```python
from build123d import *

# Parameters (mm, degrees)
RESSALTO_EXTRUS_O1_DEPTH = 3
FILETE1_SIZE             = 3.5
FILETE1_SIZE_2           = 2
ESBO_O2_R                = 0.5
RESSALTO_EXTRUS_O4_DEPTH = 0.6
ESBO_O3_R                = 0.5
RESSALTO_EXTRUS_O5_DEPTH = 0.4
FILETE2_R                = 0.2
FILETE2_OF_ESPELHAR1_R   = 0.2
ESBO_O4_R                = 0.4
CORTE_EXTRUS_O1_DEPTH    = 8.735632008


with BuildPart() as part:
    # Esboço1 → Ressalto-extrusão1 (new, symmetric)
    with BuildSketch(Plane(origin=(0, 0, 0), x_dir=(0, 0, -1), z_dir=(1, 0, 0))):
        Polygon((0, 0), (4, 0), (4, -2.8), (-3, -2.8), (-3, -1.8), (2.5, -1.8), (2.5, -1), (0, -1), align=None)
    extrude(amount=RESSALTO_EXTRUS_O1_DEPTH, both=True)

    # Filete1
    # an asymmetric fillet: 3.5, 2 mm, written as the material it takes off along each edge
    with BuildSketch(Plane(origin=(11.75, -2.8, -4), x_dir=(0, 0, 1), z_dir=(-1, 0, 0))) as filete1_piece_1:
        with BuildLine():
            Bezier((FILETE1_SIZE, 0), (0, 0), (0, FILETE1_SIZE_2), weights=[1, 0.707106781, 1])
            Line((0, FILETE1_SIZE_2), (0, 0))
            Line((0, 0), (FILETE1_SIZE, 0))
        make_face()
    extrude(amount=23.5, mode=Mode.SUBTRACT)

    # Esboço2 → Ressalto-extrusão4 (add)
    with BuildSketch(Plane(origin=(0, -1.8, 0), x_dir=(1, 0, 0), z_dir=(0, 1, 0))):
        with Locations(Location((-2, -2, 0), (0, 0, 90))):
            Circle(ESBO_O2_R)
    ressalto_extrus_o4 = extrude(amount=RESSALTO_EXTRUS_O4_DEPTH)

    # Esboço3 → Ressalto-extrusão5 (add)
    with BuildSketch(Plane.XZ.offset(1)):
        with Locations(Location((-2, -1, 0), (0, 0, 90))):
            Circle(ESBO_O3_R)
    ressalto_extrus_o5 = extrude(amount=RESSALTO_EXTRUS_O5_DEPTH)

    # Filete2
    filete2_edges = [part.edges().sort_by_distance(p)[0] for p in [
        (-2, -1.2, 2.5),
        (-2, -1.4, -1.5),
    ]]
    fillet(filete2_edges, radius=FILETE2_R)

    # Espelhar1: Ressalto-extrusão4, Ressalto-extrusão5 across plane
    add(ressalto_extrus_o4.mirror(Plane(origin=(0, 0, 0), x_dir=(0, 0, 1), z_dir=(1, 0, 0))))
    add(ressalto_extrus_o5.mirror(Plane(origin=(0, 0, 0), x_dir=(0, 0, 1), z_dir=(1, 0, 0))))

    # Filete2 of Espelhar1
    filete2_of_espelhar1_edges = [part.edges().sort_by_distance(p)[0] for p in [
        (2, -1.2, 2.5),
        (2, -1.4, -1.5),
    ]]
    fillet(filete2_of_espelhar1_edges, radius=FILETE2_OF_ESPELHAR1_R)

    # Esboço4 → Corte-extrusão1 (cut, through all)
    with BuildSketch(Plane.ZY.offset(3)):
        with Locations((-2.5, -1.4)):
            Circle(ESBO_O4_R)
    extrude(amount=-CORTE_EXTRUS_O1_DEPTH, mode=Mode.SUBTRACT)


solid = part.part
```
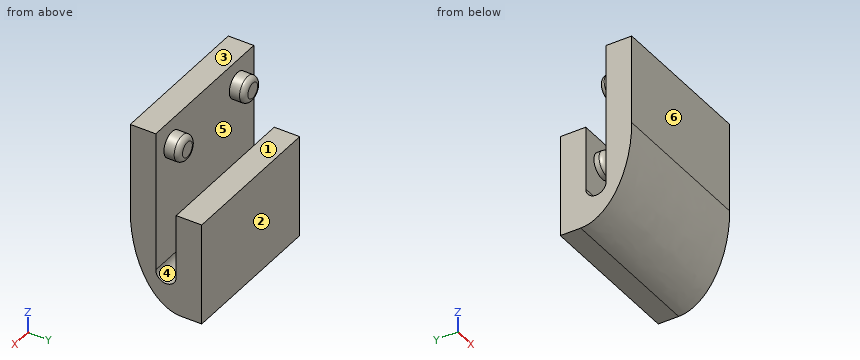
Input: part model. Units: mm. Frame: model coordinates. Face numbers are marked on the shaded views. A direction names the side the tool comes from. Coordinates: 2 decimals unless noted, no trailing zeros. Loops run counter-clockwise (first coordinate to the right, second up) from the corner with the lowest first, then second, coordinate; pieces in that order, holes last. Notation, with made-up numbers: (0.25, 35) -> (55.25, 35) arc R28 cw to (55.25, 71) -> close; hole circle Ø3 at (52.5, 25). An arc over 180 degrees is marked (long way). Use a Markdown table: item, result.
1) Contact query for flat-ended pins moving along their axis: pin 1 (0.5 mm diameter, centred on x = -2, z = -1, fed in from -Y); pin 2 (0.5 mm diameter, centred on x = 2, z = 2, fed in from +Y). Output: stop coordinate, or through.
Results found:
| item | result |
|---|---|
| pin 1 | stops at y = -2.79 |
| pin 2 | stops at y = -1.2 |
2) Access query for the marked faces 1 and 2. Directions: +Z, -Z, +X, -X, +Y, -Y. A direction counts if a zero-diameter tool reaches every point of the face in a straight line with its end or side. Return the directions, or none.
Results found:
| item | result |
|---|---|
| face 1 | +Z, +X, -X, +Y |
| face 2 | +Z, -Z, +X, -X, +Y |
3) Material intervals for line 1 along Y through (x, z) = (1.25, -0.5); line 2 along Z through (x, y) = (1.25, -0.15); line 3 along Y through (x, z) = (-1, 1.75), sorted ascending. Write a range as from..to.
Results found:
| item | result |
|---|---|
| line 1 | y = -2.8..-1.8, -1..0 |
| line 2 | z = -4..0 |
| line 3 | y = -2.8..-1.8 |
4) Cut plane A-A (z = 2). Return the cut outline in (x, y).
Results found:
| item | result |
|---|---|
| outline | (-3, -2.8) -> (3, -2.8) -> (3, -1.8) -> (2.5, -1.8) -> (2.5, -1.4) arc R0.2 ccw to (2.3, -1.2) -> (1.7, -1.2) arc R0.2 ccw to (1.5, -1.4) -> (1.5, -1.8) -> (-1.5, -1.8) -> (-1.5, -1.4) arc R0.2 ccw to (-1.7, -1.2) -> (-2.3, -1.2) arc R0.2 ccw to (-2.5, -1.4) -> (-2.5, -1.8) -> (-3, -1.8) -> close |
5) Cut plane B-B (y = -1.3). Give the number of separate pieces and of enclosed holes in the cut face, then the cut area to 3 significant figures.
Results found:
| item | result |
|---|---|
| separate pieces | 5 |
| enclosed holes | 0 |
| area | 8.82 mm2 |
6) Cut plane C-C (y = -0.45). Return the cut outline in (x, z).
Results found:
| item | result |
|---|---|
| outline | (-3, -4) -> (3, -4) -> (3, 0) -> (-3, 0) -> close |
7) Pull-direction query (Y, two-part tool) for the marked faces 3, 4, 5 and 6; classes: released by +Y, released by -Y, zero draft, split by the parting line, or undercut.
Results found:
| item | result |
|---|---|
| face 3 | zero draft |
| face 4 | undercut |
| face 5 | undercut |
| face 6 | released by -Y |
